```python
from build123d import *

# Parameters (mm, degrees)
EXTRUDE_1_OUTLINE_R       = 27.5
EXTRUDE_1_DEPTH           = 6
SKETCH_2_R                = 6
CUT_EXTRUDE_1_DEPTH       = 4
SKETCH_3_R                = 4
CUT_EXTRUDE_2_DEPTH       = 40.096035605
PATTERN_CIRCULAR_1_COUNT  = 6
SKETCH_4_R                = 15
EXTRUDE_2_DEPTH           = 16
MIRROR_1_COPY_1_SKETCH_R  = 6
MIRROR_1_COPY_1_DEPTH     = 4
MIRROR_1_COPY_2_SKETCH_R  = 6
MIRROR_1_COPY_2_DEPTH     = 4
MIRROR_1_COPY_3_SKETCH_R  = 6
MIRROR_1_COPY_3_DEPTH     = 4
MIRROR_1_COPY_4_SKETCH_R  = 6
MIRROR_1_COPY_4_DEPTH     = 4
MIRROR_1_COPY_5_SKETCH_R  = 6
MIRROR_1_COPY_5_DEPTH     = 4
MIRROR_1_COPY_6_SKETCH_R  = 4
MIRROR_1_COPY_6_DEPTH     = 40.096035605
MIRROR_1_COPY_7_SKETCH_R  = 4
MIRROR_1_COPY_7_DEPTH     = 40.096035605
MIRROR_1_COPY_8_SKETCH_R  = 4
MIRROR_1_COPY_8_DEPTH     = 40.096035605
MIRROR_1_COPY_9_SKETCH_R  = 4
MIRROR_1_COPY_9_DEPTH     = 40.096035605
MIRROR_1_COPY_10_SKETCH_R = 4
MIRROR_1_COPY_10_DEPTH    = 40.096035605
CUT_EXTRUDE_3_DEPTH       = 48.921811318
CHAMFER_1_SIZE            = 0.3
SKETCH_7_W                = 1.65
SKETCH_7_H                = 28.065698604


# Read off the part's stored shape, not the designer's step: 凸台-拉伸1
with BuildPart() as part:
    # 凸台-拉伸1 outline → 凸台-拉伸1 (new body)
    with BuildSketch(Plane.XY):
        Circle(EXTRUDE_1_OUTLINE_R)
    extrude_1 = extrude(amount=EXTRUDE_1_DEPTH)

    # 草图2 → 切除-拉伸1 (cut)
    with BuildSketch(Plane.XY.offset(6)):
        with Locations((0, 20)):
            Circle(SKETCH_2_R)
    cut_extrude_1 = extrude(amount=-CUT_EXTRUDE_1_DEPTH, mode=Mode.SUBTRACT)

    # 草图3 → 切除-拉伸2 (cut, through all)
    with BuildSketch(Plane.XY.offset(2)):
        with Locations((0, 20)):
            Circle(SKETCH_3_R)
    cut_extrude_2 = extrude(amount=-CUT_EXTRUDE_2_DEPTH, mode=Mode.SUBTRACT)

    # 阵列(圆周)1: 切除-拉伸1, 切除-拉伸2 ×6 about axis
    pattern_circular_1_axis = Axis((0, 0, 0), (0, 0, 1))
    add([cut_extrude_1.rotate(pattern_circular_1_axis, i * 360 / PATTERN_CIRCULAR_1_COUNT) for i in range(1, PATTERN_CIRCULAR_1_COUNT)], mode=Mode.SUBTRACT)
    add([cut_extrude_2.rotate(pattern_circular_1_axis, i * 360 / PATTERN_CIRCULAR_1_COUNT) for i in range(1, PATTERN_CIRCULAR_1_COUNT)], mode=Mode.SUBTRACT)

    # 草图4 → 凸台-拉伸2 (add)
    with BuildSketch(Plane(origin=(0, 0, 0), x_dir=(-1, 0, 0), z_dir=(0, 0, -1))):
        with Locations(Location((0, 0, 0), (0, 0, 180))):
            Circle(SKETCH_4_R)
    extrude(amount=EXTRUDE_2_DEPTH)

    # 镜向1: 凸台-拉伸1, 切除-拉伸1, 切除-拉伸2 across plane
    add(extrude_1.mirror(Plane(origin=(0, 0, -8), x_dir=(1, 0, 0), z_dir=(0, 0, -1))))
    add(cut_extrude_1.mirror(Plane(origin=(0, 0, -8), x_dir=(1, 0, 0), z_dir=(0, 0, -1))), mode=Mode.SUBTRACT)
    add(cut_extrude_2.mirror(Plane(origin=(0, 0, -8), x_dir=(1, 0, 0), z_dir=(0, 0, -1))), mode=Mode.SUBTRACT)

    # 镜向1 copy 1 sketch → 镜向1 copy 1 (cut)
    with BuildSketch(Plane(origin=(0, 0, -22), x_dir=(0.5000000000000001, 0.8660254037844386, 0), z_dir=(0, 0, -1))):
        with Locations((0, -20)):
            Circle(MIRROR_1_COPY_1_SKETCH_R)
    extrude(amount=-MIRROR_1_COPY_1_DEPTH, mode=Mode.SUBTRACT)

    # 镜向1 copy 2 sketch → 镜向1 copy 2 (cut)
    with BuildSketch(Plane(origin=(0, 0, -22), x_dir=(-0.4999999999999998, 0.8660254037844387, 0), z_dir=(0, 0, -1))):
        with Locations((0, -20)):
            Circle(MIRROR_1_COPY_2_SKETCH_R)
    extrude(amount=-MIRROR_1_COPY_2_DEPTH, mode=Mode.SUBTRACT)

    # 镜向1 copy 3 sketch → 镜向1 copy 3 (cut)
    with BuildSketch(Plane(origin=(0, 0, -22), x_dir=(-1, 0, 0), z_dir=(0, 0, -1))):
        with Locations((0, -20)):
            Circle(MIRROR_1_COPY_3_SKETCH_R)
    extrude(amount=-MIRROR_1_COPY_3_DEPTH, mode=Mode.SUBTRACT)

    # 镜向1 copy 4 sketch → 镜向1 copy 4 (cut)
    with BuildSketch(Plane(origin=(0, 0, -22), x_dir=(-0.5000000000000004, -0.8660254037844384, 0), z_dir=(0, 0, -1))):
        with Locations((0, -20)):
            Circle(MIRROR_1_COPY_4_SKETCH_R)
    extrude(amount=-MIRROR_1_COPY_4_DEPTH, mode=Mode.SUBTRACT)

    # 镜向1 copy 5 sketch → 镜向1 copy 5 (cut)
    with BuildSketch(Plane(origin=(0, 0, -22), x_dir=(0.5000000000000001, -0.8660254037844386, 0), z_dir=(0, 0, -1))):
        with Locations((0, -20)):
            Circle(MIRROR_1_COPY_5_SKETCH_R)
    extrude(amount=-MIRROR_1_COPY_5_DEPTH, mode=Mode.SUBTRACT)

    # 镜向1 copy 6 sketch → 镜向1 copy 6 (cut, through all)
    with BuildSketch(Plane(origin=(0, 0, -18), x_dir=(0.5000000000000001, 0.8660254037844386, 0), z_dir=(0, 0, -1))):
        with Locations((0, -20)):
            Circle(MIRROR_1_COPY_6_SKETCH_R)
    extrude(amount=-MIRROR_1_COPY_6_DEPTH, mode=Mode.SUBTRACT)

    # 镜向1 copy 7 sketch → 镜向1 copy 7 (cut, through all)
    with BuildSketch(Plane(origin=(0, 0, -18), x_dir=(-0.4999999999999998, 0.8660254037844387, 0), z_dir=(0, 0, -1))):
        with Locations((0, -20)):
            Circle(MIRROR_1_COPY_7_SKETCH_R)
    extrude(amount=-MIRROR_1_COPY_7_DEPTH, mode=Mode.SUBTRACT)

    # 镜向1 copy 8 sketch → 镜向1 copy 8 (cut, through all)
    with BuildSketch(Plane(origin=(0, 0, -18), x_dir=(-1, 0, 0), z_dir=(0, 0, -1))):
        with Locations((0, -20)):
            Circle(MIRROR_1_COPY_8_SKETCH_R)
    extrude(amount=-MIRROR_1_COPY_8_DEPTH, mode=Mode.SUBTRACT)

    # 镜向1 copy 9 sketch → 镜向1 copy 9 (cut, through all)
    with BuildSketch(Plane(origin=(0, 0, -18), x_dir=(-0.5000000000000004, -0.8660254037844384, 0), z_dir=(0, 0, -1))):
        with Locations((0, -20)):
            Circle(MIRROR_1_COPY_9_SKETCH_R)
    extrude(amount=-MIRROR_1_COPY_9_DEPTH, mode=Mode.SUBTRACT)

    # 镜向1 copy 10 sketch → 镜向1 copy 10 (cut, through all)
    with BuildSketch(Plane(origin=(0, 0, -18), x_dir=(0.5000000000000001, -0.8660254037844386, 0), z_dir=(0, 0, -1))):
        with Locations((0, -20)):
            Circle(MIRROR_1_COPY_10_SKETCH_R)
    extrude(amount=-MIRROR_1_COPY_10_DEPTH, mode=Mode.SUBTRACT)

    # 草图5 → 切除-拉伸3 (cut, through all)
    with BuildSketch(Plane.XY.offset(6)):
        with BuildLine():
            Line((6.915063509, 6.977241336), (2.584936491, 9.477241336))
            Line((2.584936491, 9.477241336), (1.370470396, 7.373724357))
            ThreePointArc((1.370470396, 7.373724357), (-3.75, -6.495190528), (5.700597415, 4.873724357))
            Line((5.700597415, 4.873724357), (6.915063509, 6.977241336))
        make_face()
    extrude(amount=-CUT_EXTRUDE_3_DEPTH, mode=Mode.SUBTRACT)

    # 倒角1
    chamfer_1_edges = [part.edges().sort_by_distance(p)[0] for p in [
        (-27.5, 0, 0),
        (-27.5, 0, 6),
        (-27.5, 0, -16),
        (-27.5, 0, -22),
    ]]
    chamfer(chamfer_1_edges, length=CHAMFER_1_SIZE)

    # 草图7 → M4 螺纹孔1 (revolve, cut)
    with BuildSketch(Plane(origin=(4.75, 8.227241336, -8.001910076), x_dir=(0.866025403784438, -0.5000000000000012, 0), z_dir=(0, 0, 1))):
        with Locations((0.825, 14.032849302)):
            Rectangle(SKETCH_7_W, SKETCH_7_H)
    revolve(axis=Axis((1.575, 2.727980022, -8.001910076), (0.5000000000000012, 0.8660254037844379, 0)), mode=Mode.SUBTRACT)


solid = part.part
```
Could you check a few things on this model? Use its own coordinates, in mm. A direction names the side the tool comes from. Give positions to 0.01 mm unless a question says otherwise; leave off trailing zeros. Loops run counter-clockwise (first coordinate to the right, second up) from the corner with the lowest first, then second, coordinate; pieces in that order, holes last. Notation, with made-up numbers: (16, 46) -> (26, 46) arc R14 cw to (26, 55) -> close; hole circle Ø11 at (2.5, -39). An arc over 180 degrees is marked (long way). Put each result on its own line as item: value.
(1) For faces 3 (the face through (6.7, 7.1, -7.8)), 4 (the face through (-12.56, 13.65, 4.03)), 5 (the face through (-11.056, -10.138, -7.888)), 6 (the face through (0.78, -14.05, -20.03)), which set-ups out of +Z, -Z, +X, -X, +Y, -Y let a thin tool reach every point of the face, with its end or its side?
Computed:
face 3: +Z, -Z
face 4: +Z
face 5: none
face 6: -Z
(2) I'm going to push flat-ended pins straight in: pin 1 Ø4 at (x, z) = (2.5, 3) entering from +Y; pin 2 Ø9 at (x, y) = (0, 20) entering from +Z; pin 3 Ø8 at (x, z) = (6.5, -7.5) entering from -Y. Where does each tip first touch, or does it pass through?
Computed:
pin 1: y = 27.5
pin 2: z = 2
pin 3: y = -14.79
(3) Imagine slicing it at A-A on y = 0. Write out the boundary of the cut face in (x, z).
Computed:
outline: (-27.5, -21.7) -> (-27.2, -22) -> (-7.5, -22) -> (-7.5, 6) -> (-27.2, 6) -> (-27.5, 5.7) -> (-27.5, 0.3) -> (-27.2, 0) -> (-15, 0) -> (-15, -16) -> (-27.2, -16) -> (-27.5, -16.3) -> close; (7.5, -22) -> (27.2, -22) -> (27.5, -21.7) -> (27.5, -16.3) -> (27.2, -16) -> (15, -16) -> (15, 0) -> (27.2, 0) -> (27.5, 0.3) -> (27.5, 5.7) -> (27.2, 6) -> (7.5, 6) -> close
(4) Please list where these lines run through material, in increasing order: probe 1 along Y at (x, z) = (0, -19.8); probe 2 along Y at (x, z) = (0, -16.95); probe 3 along Z at (x, y) = (15.5, 16.5). Write a range as [from, to].
Computed:
probe 1: [-27.5, -26], [-14, -7.5], [7.5, 14], [26, 27.5]
probe 2: [-27.5, -24], [-16, -7.5], [7.5, 16], [24, 27.5]
probe 3: [-22, -16], [0, 6]
(5) Imagine slicing it at C-C on x = 0. State how many separate pieces and enclosed holes the cut face has, plus the area to 3 significant figures.
Computed:
separate pieces: 6
enclosed holes: 0
area: 464 mm^2
(6) Imagine slicing it at B-B on z = -1.75. Write out the boundary of the cut face in (x, y).
Computed:
outline: circle Ø30 at (0, 0); hole (1.37, 7.37) arc R7.5 ccw (long way) to (5.7, 4.87) -> (6.92, 6.98) -> (2.58, 9.48) -> close
(7) Thinking about a two-plate mould opening in X: for faces 1 (the face through (20.4, 7.2, -18)), 2 (the face through (-5.961, -26.846, 2.962)), which applies, pulls with the +X half, pulls with the -X half, needs draft (parallel to the pull), parting line crosses it, or undercut?
Computed:
face 1: undercut
face 2: parting line crosses it
